Can you work these out from the drawing? Everything is in mm from the part's minimum corner. Coordinates: 2 decimals unless noted, no trailing zeros. Loops run counter-clockwise (first coordinate to the right, second up) from the corner with the lowest first, then second, coordinate; pieces in that order, holes last. Notation, with made-up numbers: (37, -9.75) - (96, -9.75) arc R26 cw to (96, 8.25) - close; hole circle Ø11 at (-15, 23.25). An arc over 180 degrees is marked (long way). Put each result on its own line as item: value. Start each with the question number.
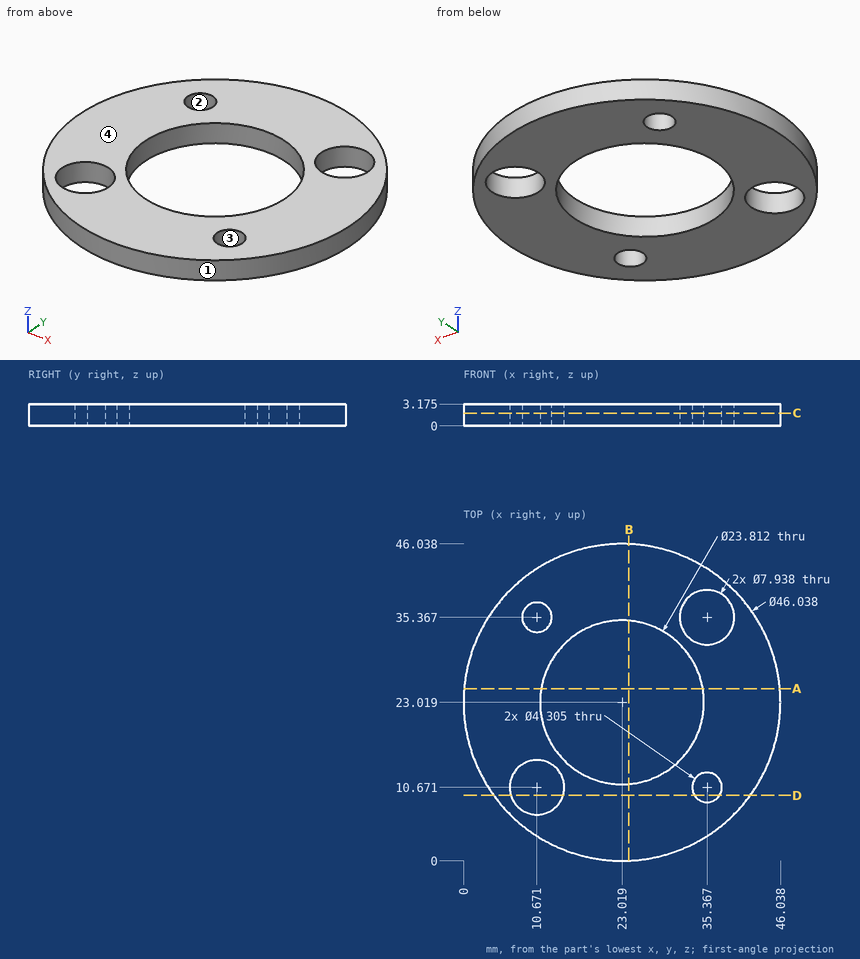
Q1. I want a section at C-C on z = 1.85. List the corners of the cut face in (x, y) for me (1 decimal).
Q2. I want a section at D-D on y = 9.5. Count the separate pieces of the cut face and the enclosed holes in it.
Q3. I want a section at B-B on x = 24. List the corners of the cut face in (y, z) for me (1 decimal).
Q4. Will these pins go through, and if not, where does the flat tip stop? pin 1 (1.5 mm diameter, centred on x = 22.5, z = 0.5, fed in from +Y); pin 2 (1 mm diameter, centred on x = 30.5, z = 2, fed in from -Y) (1 decimal).
Q5. I want a section at A-A on y = 25. List the corners of the cut face in (x, z) for me (1 decimal).
Q6. We'd pull the mould along Y, two halves only. Please class the marked faces 1, 2, 3 and 4: released by +Y, released by -Y, zero draft, split by the parting line, or undercut.
Q7. Please list where these lines run through material, in increasing order: line 1 along X through (y, z) = (12, 1.55) (1 decimal); line 2 along Y through (x, z) = (23.5, 0.25) (1 decimal); line 3 along Y through (x, z) = (20.5, 2.35) (1 decimal). Write a range as [from, to].
Calculated:
1. outline: circle Ø46 at (23, 23); hole circle Ø7.9 at (10.7, 10.7); hole circle Ø4.3 at (10.7, 35.4); hole circle Ø23.8 at (23, 23); hole circle Ø7.9 at (35.4, 35.4); hole circle Ø4.3 at (35.4, 10.7)
2. separate pieces: 3
2. enclosed holes: 0
3. outline: (0, 0) - (11.2, 0) - (11.2, 3.2) - (0, 3.2) - close; (34.9, 0) - (46, 0) - (46, 3.2) - (34.9, 3.2) - close
4. pin 1: y = 46.04
4. pin 2: y = 1.1
5. outline: (0.1, 0) - (11.3, 0) - (11.3, 3.2) - (0.1, 3.2) - close; (34.8, 0) - (46, 0) - (46, 3.2) - (34.8, 3.2) - close
6. face 1: split by the parting line
6. face 2: undercut
6. face 3: undercut
6. face 4: zero draft
7. line 1: [2.8, 6.9], [14.4, 18.5], [27.5, 33.7], [37.1, 43.2]
7. line 2: [0, 11.1], [34.9, 46]
7. line 3: [0.1, 11.4], [34.7, 45.9]
